Part model, mm, in its own coordinate system. Round coordinates to 2 decimals unless told otherwise and drop trailing zeros. Loops run counter-clockwise (first coordinate to the right, second up) from the corner with the lowest first, then second, coordinate; pieces in that order, holes last. Notation, with made-up numbers: M -4.75,22 L 45.25,22 A22 cw 45.25,47 Z; hole C 81,-20 d7. An arc over 180 degrees is marked long. Write each question's results on one line, items separated by ' | '.
from build123d import *

# Parameters (mm, degrees)
SKETCH1_R               = 49.53
SKETCH1_R_2             = 46.99
BOSS_EXTRUDE1_DEPTH     = 182.88
CUT_EXTRUDE1_DEPTH      = 177.8
SKETCH3_R               = 49.53
SKETCH3_R_2             = 46.99
BOSS_EXTRUDE2_DEPTH     = 2.54
SKETCH4_R               = 49.53
SKETCH4_R_2             = 46.99
BOSS_EXTRUDE3_DEPTH     = 2.54
BOSS_EXTRUDE4_START     = -5.08
SKETCH5_R               = 49.53
BOSS_EXTRUDE4_DEPTH     = 5.08
SKETCH6_W               = 50.419
SKETCH6_H               = 4.699
BOSS_EXTRUDE5_DEPTH     = 2.54
SKETCH7_R               = 0.8255
BOSS_EXTRUDE6_DEPTH     = 2.54
CIRPATTERN2_COUNT       = 8
CUT_EXTRUDE2_DEPTH      = 199.209531052
CUT_EXTRUDE2_DEPTH_BACK = 199.209531052
SKETCH8_W               = 132.398464635
SKETCH8_H               = 191.049097361


with BuildPart() as part:
    # Sketch1 → Boss-Extrude1 (new, symmetric)
    with BuildSketch(Plane(origin=(0, 0, 0), x_dir=(1, 0, 0), z_dir=(0, 1, 0))):
        with Locations(Location((0, 0, 0), (0, 0, 270))):
            Circle(SKETCH1_R)
        with Locations(Location((0, 0, 0), (0, 0, 270))):
            Circle(SKETCH1_R_2, mode=Mode.SUBTRACT)
    extrude(amount=BOSS_EXTRUDE1_DEPTH, both=True)

    # Sketch2 → Cut-Extrude1 (cut, symmetric)
    with BuildSketch(Plane(origin=(0, 0, 0), x_dir=(1, 0, 0), z_dir=(0, 1, 0))):
        with BuildLine():
            Line((34.339077963, -32.07628134), (36.13611782, -33.873321197))
            ThreePointArc((36.13611782, -33.873321197), (45.710930003, -19.071753413), (49.49527883, -1.854258207))
            Line((49.49527883, -1.854258207), (46.953400585, -1.854258207))
            ThreePointArc((46.953400585, -1.854258207), (43.364264524, -18.099742051), (34.339077963, -32.07628134))
        make_face()
        with BuildLine():
            ThreePointArc((1.584890151, -49.504636381), (18.664975227, -45.878530924), (33.425440685, -36.550797734))
            Line((33.425440685, -36.550797734), (31.627502039, -34.752859088))
            ThreePointArc((31.627502039, -34.752859088), (17.692915235, -43.531837205), (1.584890151, -46.963264614))
            Line((1.584890151, -46.963264614), (1.584890151, -49.504636381))
        make_face()
        with BuildLine():
            ThreePointArc((-33.543952964, -36.442065248), (-19.03558139, -45.726005086), (-2.225109849, -49.479993797))
            Line((-2.225109849, -49.479993797), (-2.225109849, -46.937287801))
            ThreePointArc((-2.225109849, -46.937287801), (-18.063572268, -43.379343666), (-31.746279167, -34.644391451))
            Line((-31.746279167, -34.644391451), (-33.543952964, -36.442065248))
        make_face()
        with BuildLine():
            Line((46.949282998, 1.955741793), (49.491372723, 1.955741793))
            ThreePointArc((49.491372723, 1.955741793), (45.777644234, 18.911059948), (36.442065248, 33.543952964))
            Line((36.442065248, 33.543952964), (34.644391451, 31.746279167))
            ThreePointArc((34.644391451, 31.746279167), (43.430990742, 17.93903964), (46.949282998, 1.955741793))
        make_face()
        with BuildLine():
            ThreePointArc((-49.49527883, -1.854258207), (-45.741824116, -18.997537381), (-36.245883162, -33.755841773))
            Line((-36.245883162, -33.755841773), (-34.448634556, -31.958593167))
            ThreePointArc((-34.448634556, -31.958593167), (-43.39516767, -18.025524205), (-46.953400585, -1.854258207))
            Line((-46.953400585, -1.854258207), (-49.49527883, -1.854258207))
        make_face()
        with BuildLine():
            Line((31.958593167, 34.448634556), (33.755841773, 36.245883162))
            ThreePointArc((33.755841773, 36.245883162), (18.873008967, 45.79334485), (1.584890151, 49.504636381))
            Line((1.584890151, 49.504636381), (1.584890151, 46.963264614))
            ThreePointArc((1.584890151, 46.963264614), (17.900986276, 43.446689061), (31.958593167, 34.448634556))
        make_face()
        with BuildLine():
            ThreePointArc((-36.550797734, 33.425440685), (-45.80828813, 18.836709868), (-49.491372723, 1.955741793))
            Line((-49.491372723, 1.955741793), (-46.949282998, 1.955741793))
            ThreePointArc((-46.949282998, 1.955741793), (-43.461630715, 17.864678995), (-34.752859088, 31.627502039))
            Line((-34.752859088, 31.627502039), (-36.550797734, 33.425440685))
        make_face()
        with BuildLine():
            Line((-2.225109849, 46.937287801), (-2.225109849, 49.479993797))
            ThreePointArc((-2.225109849, 49.479993797), (-19.242893169, 45.63914945), (-33.873321197, 36.13611782))
            Line((-33.873321197, 36.13611782), (-32.07628134, 34.339077963))
            ThreePointArc((-32.07628134, 34.339077963), (-18.270880717, 43.292436035), (-2.225109849, 46.937287801))
        make_face()
    extrude(amount=CUT_EXTRUDE1_DEPTH, both=True, mode=Mode.SUBTRACT)

    # Sketch3 → Boss-Extrude2 (add, symmetric)
    with BuildSketch(Plane(origin=(0, 91.44, 0), x_dir=(1, 0, 0), z_dir=(0, 1, 0))):
        with Locations(Location((0, 0, 0), (0, 0, 270))):
            Circle(SKETCH3_R)
        with Locations(Location((0, 0, 0), (0, 0, 270))):
            Circle(SKETCH3_R_2, mode=Mode.SUBTRACT)
    boss_extrude2 = extrude(amount=BOSS_EXTRUDE2_DEPTH, both=True)

    # Mirror1: Boss-Extrude2 across plane
    add(boss_extrude2.mirror(Plane.ZX))

    # Sketch4 → Boss-Extrude3 (add, symmetric)
    with BuildSketch(Plane(origin=(0, 0, 0), x_dir=(1, 0, 0), z_dir=(0, 1, 0))):
        with Locations(Location((0, 0, 0), (0, 0, 270))):
            Circle(SKETCH4_R)
        with Locations(Location((0, 0, 0), (0, 0, 270))):
            Circle(SKETCH4_R_2, mode=Mode.SUBTRACT)
    extrude(amount=BOSS_EXTRUDE3_DEPTH, both=True)

    # Sketch5 → Boss-Extrude4 (add)
    with BuildSketch(Plane.XZ.offset(182.88).offset(BOSS_EXTRUDE4_START)):
        with Locations(Location((0, 0, 0), (0, 0, 90))):
            Circle(SKETCH5_R)
    extrude(amount=BOSS_EXTRUDE4_DEPTH)

    # Sketch6 → Boss-Extrude5 (add)
    with BuildSketch(Plane(origin=(0, -177.8, 0), x_dir=(1, 0, 0), z_dir=(0, 1, 0))):
        Rectangle(SKETCH6_W, SKETCH6_H)
    extrude(amount=BOSS_EXTRUDE5_DEPTH)

    # Sketch7 → Boss-Extrude6 (add)
    with BuildSketch(Plane(origin=(0, 182.88, 0), x_dir=(1, 0, 0), z_dir=(0, 1, 0))):
        with Locations(Location((48.26, 0, 0), (0, 0, 270))):
            Circle(SKETCH7_R)
    boss_extrude6 = extrude(amount=BOSS_EXTRUDE6_DEPTH)

    # CirPattern2: Boss-Extrude6 ×8 about axis
    cirpattern2_axis = Axis((0, 0, 0), (0, 1, 0))
    for i in range(1, CIRPATTERN2_COUNT):
        add(boss_extrude6.rotate(cirpattern2_axis, i * 360 / CIRPATTERN2_COUNT))

    # Sketch8 → Cut-Extrude2 (cut, two sides: drawn at the far end of the back side and taken through both)
    with BuildSketch(Plane(origin=(0, 0, 0), x_dir=(0, 0, -1), z_dir=(1, 0, 0)).offset(-CUT_EXTRUDE2_DEPTH_BACK)):
        with Locations((2.481127426, -95.524548681)):
            Rectangle(SKETCH8_W, SKETCH8_H)
    extrude(amount=CUT_EXTRUDE2_DEPTH + CUT_EXTRUDE2_DEPTH_BACK, mode=Mode.SUBTRACT)


solid = part.part
Item 1: Band-saw the part on C-C on x = -5. Give the cut face in (y, z).
Filled sheet:
outline: M 0,-49.28 L 2.54,-49.28 L 2.54,-46.72 L 0,-46.72 Z; M 0,46.72 L 2.54,46.72 L 2.54,49.28 L 0,49.28 Z; M 88.9,-49.28 L 93.98,-49.28 L 93.98,-46.72 L 88.9,-46.72 Z; M 88.9,46.72 L 93.98,46.72 L 93.98,49.28 L 88.9,49.28 Z; M 177.8,-49.28 L 182.88,-49.28 L 182.88,-46.72 L 177.8,-46.72 Z; M 177.8,46.72 L 182.88,46.72 L 182.88,49.28 L 177.8,49.28 Z
Item 2: Band-saw the part on B-B on z = 25. Give the cut face in (x, y), and give its area (3 significant figures).
Filled sheet:
outline: M -42.76,0 L -39.79,0 L -39.79,2.54 L -42.76,2.54 Z; M -42.76,88.9 L -39.79,88.9 L -39.79,93.98 L -42.76,93.98 Z; M -42.76,177.8 L -39.79,177.8 L -39.79,182.88 L -42.76,182.88 Z; M 39.79,0 L 42.76,0 L 42.76,2.54 L 39.79,2.54 Z; M 39.79,88.9 L 42.76,88.9 L 42.76,93.98 L 39.79,93.98 Z; M 39.79,177.8 L 42.76,177.8 L 42.76,182.88 L 39.79,182.88 Z | area: 75.4 mm^2
Item 3: Wall check: L1, parallel to Y at x = 23, z = -42; L2, parallel to X at y = 131, z = 0; L3, parallel to X at y = 150, z = 34. Give the ranges that are in metal, low to high.
Filled sheet:
L1: 0 to 2.54, 88.9 to 93.98, 177.8 to 182.88 | L2: -49.53 to -46.99, 46.99 to 49.53 | L3: -36.02 to -32.44, 32.44 to 36.02
Item 4: Band-saw the part on A-A on y = 152.5. Count the separate pieces of the cut face and the enclosed holes in it, and give its area (3 significant figures).
Filled sheet:
separate pieces: 8 | enclosed holes: 0 | area: 77.4 mm^2
Item 5: Drop flat-ended pins along their axis: P1, Ø4.5, axis at x = -44, z = -20, coming from the +Y side; P2, Ø5, axis at x = -39.5, z = 37.5, coming from the -Y side; P3, Ø3, axis at y = 143, z = -47.5, coming from the -X side; P4, Ø3, axis at x = 35, y = 107, coming from the +Z side. Give the stop position or say it passes through.
Filled sheet:
P1: y = 182.88 | P2: through | P3: x = -2.23 | P4: z = 36.48
